Geometry check sheet. Reference: the model listing, model coordinates, mm. A direction names the side the tool comes from. Coordinates: 2 decimals unless noted, no trailing zeros. Loops run counter-clockwise (first coordinate to the right, second up) from the corner with the lowest first, then second, coordinate; pieces in that order, holes last. Notation, with made-up numbers: (74, 47) - (133, 47) arc R13 ccw to (133, 64) - close; hole circle Ø8 at (66, 69). An arc over 180 degrees is marked (long way). One line per item, written item: value.
from build123d import *

# Parameters (mm, degrees)
F0_W     = 71.088023
F0_H     = 3.453668
F0_W_2   = 70.599534
F0_H_2   = 3.316156
F0_W_3   = 70.224609
F0_H_3   = 4.029283
F0_W_4   = 70.512414
F0_H_4   = 4.029279
F0_W_5   = 70.800219
F0_H_5   = 3.453669
F0_W_6   = 70.994157
F0_H_6   = 3.551615
F0_W_7   = 72.216179
F0_H_7   = 3.354305
F0_W_8   = 72.610803
F0_H_8   = 2.762366
F0_W_9   = 73.005423
F0_H_9   = 3.354303
F0_W_10  = 72.808113
F0_H_10  = 3.354299
F1_DEPTH = 3


with BuildPart() as f1:
    # F0 (on Front) → F1 (new body)
    with BuildSketch(Plane.XZ):
        Polygon((52.176289, 64.601567), (-53.791832, 64.601567), (-53.791832, 59.431892), (-8.49027, 59.431892), (-8.49027, 55.97822), (-53.791832, 55.97822), (-53.791832, 47.354873), (-8.385758, 47.354873), (-8.385758, 44.197883), (-53.791832, 44.197883), (-53.791832, 36.305401), (-8.385758, 36.305401), (-8.385758, 33.345722), (-53.791832, 33.345722), (-53.791832, 25.847867), (-7.991134, 25.847867), (-7.991134, 22.888189), (-53.791832, 22.888189), (-53.791832, 14.798397), (-7.596511, 14.798397), (-7.793822, 11.246782), (-53.791832, 11.246782), (-53.791832, 3.597572), (-8.202464, 3.597572), (-8.202464, 0), (-53.791832, 0), (-53.791832, -9.641493), (-7.914659, -9.641493), (-7.914659, -13.382968), (-53.791832, -13.382968), (-53.791832, -24.031783), (-7.914659, -24.031783), (-7.914659, -27.485449), (-53.791832, -27.485449), (-53.791832, -38.134262), (-8.202464, -38.134262), (-8.202464, -42.163543), (-53.791832, -42.163543), (-53.791832, -53.076919), (-8.202464, -53.076919), (-8.202464, -56.348752), (-53.791832, -56.348752), (-53.791832, -70.533961), (52.176289, -70.533961), (52.176289, -56.036595), (11.206436, -56.036595), (11.206436, -53.076919), (52.176289, -53.076919), (52.176289, -42.163543), (11.206436, -42.163543), (11.080521, -38.134262), (52.176289, -38.134262), (52.176289, -28.348867), (6.475631, -28.348867), (6.475631, -24.031783), (52.176289, -24.031783), (52.176289, -13.382968), (6.475631, -13.382968), (6.475631, -9.641493), (52.176289, -9.641493), (52.176289, 0), (6.763437, 0), (6.475631, 3.597572), (52.176289, 3.597572), (52.176289, 11.444095), (6.412639, 11.444095), (6.412639, 14.798397), (52.176289, 14.798397), (52.176289, 22.690875), (6.215328, 22.690875), (6.215328, 25.847867), (52.176289, 25.847867), (52.176289, 33.345722), (6.215328, 33.345722), (6.215328, 36.305401), (52.176289, 36.305401), (52.176289, 44.000566), (6.018014, 44.000566), (6.018014, 47.354873), (52.176289, 47.354873), (52.176289, 55.97822), (5.900018, 55.97822), (5.900018, 59.431892), (52.176289, 59.431892), align=None)
        with Locations((1.151222, -61.158726)):
            Rectangle(F0_W, F0_H, mode=Mode.SUBTRACT)
        with Locations((0.906978, -47.27529)):
            Rectangle(F0_W_2, F0_H_2, mode=Mode.SUBTRACT)
        with Locations((0.719515, -33.241566)):
            Rectangle(F0_W_3, F0_H_3, mode=Mode.SUBTRACT)
        with Locations((0.863418, -19.714693)):
            Rectangle(F0_W_4, F0_H_4, mode=Mode.SUBTRACT)
        with Locations((1.00732, -4.173183)):
            Rectangle(F0_W_5, F0_H_5, mode=Mode.SUBTRACT)
        with Locations((1.10429, 7.695167)):
            Rectangle(F0_W_6, F0_H_6, mode=Mode.SUBTRACT)
        with Locations((0.690593, 18.448668)):
            Rectangle(F0_W_7, F0_H_7, mode=Mode.SUBTRACT)
        with Locations((0.887905, 29.202171)):
            Rectangle(F0_W_8, F0_H_8, mode=Mode.SUBTRACT)
        with Locations((1.085214, 40.350296)):
            Rectangle(F0_W_9, F0_H_9, mode=Mode.SUBTRACT)
        with Locations((0.98656, 51.202455)):
            Rectangle(F0_W_10, F0_H_10, mode=Mode.SUBTRACT)
    extrude(amount=F1_DEPTH)


solid = f1.part
(1) Cross-section at B-B on x = -13.5. State how many separate pieces and enclosed holes the cut face has, and give its area (3 significant figures).
Reply:
separate pieces: 21
enclosed holes: 0
area: 199 mm2
(2) Access from +Z, -Z, +X, -X, +Y, -Y to the whole of each face (thin tool, end or side, straight path). Record for faces 1 (the face through (29, -1, 55.978)), 2 (the face through (52.176, -1, -19)), 3 (the face through (1, -1, -2.446)), 4 (the face through (-31, -1, -42.164)).
Reply:
face 1: +X, +Y, -Y
face 2: +Z, -Z, +X, +Y, -Y
face 3: +Y, -Y
face 4: -X, +Y, -Y
(3) Material ranges on probe 1 along X at (y, z) = (-0.8, -20); probe 2 along X at (y, z) = (-2.6, -32); probe 3 along X at (y, z) = (-2.55, -40), recorded low to high. Write a range as from..to.
Reply:
probe 1: -53.79..-34.39, 36.12..52.18
probe 2: -53.79..-34.39, 35.83..52.18
probe 3: -8.2..11.14
(4) Release check for a two-part mould opening along Z. For faces 5 (the face through (-53.792, -1, -5)), 6 (the face through (36.407, -1, -4)), 7 (the face through (-34.393, -1, -61)) record: pulls with the +Z half, pulls with the -Z half, needs draft (parallel to the pull), parting line crosses it, or undercut.
Reply:
face 5: needs draft
face 6: undercut
face 7: undercut
(5) Cross-section at A-A on z = -19.5. Record the cut outline in (x, y), and give its area (3 significant figures).
Reply:
outline: (-53.79, -3) - (-34.39, -3) - (-34.39, 0) - (-53.79, 0) - close; (36.12, -3) - (52.18, -3) - (52.18, 0) - (36.12, 0) - close
area: 106 mm2
(6) Go/stop test with a flat-tipped pin: pin 1 Ø1.5 at (y, z) = (-2, 24) entering from -X. Record where the tip stops, or that it passes through.
Reply:
pin 1: x = -7.99
